Can you work these out from the model? Positions are in its coordinate system, mm. Face numbers are marked on the shaded views. Coordinates: 2 decimals unless noted, no trailing zeros. Order: outer loops, then holes, each group sorted by start corner. A loop starts at its lowest first (then second) coordinate and runs counter-clockwise, first axis right, second up. Notation, with made-up numbers: (-37.75, 32) - (21.25, 32) arc R31 ccw to (21.25, 59) - close; hole circle Ø11 at (21, -39.5). An arc over 180 degrees is marked (long way). Use a Markdown table: item, result. Add a question column.
(1) For pin 1 Ø2 at (y, z) = (14, 3) entering from -X; pin 2 Ø1.5 at (x, z) = (-14.5, 9) entering from +Y; pin 3 Ø1 at (y, z) = (25, 1.5) entering from +X; pin 4 Ø6 at (x, y) = (-40, 0) entering from +Z, each with a flat end and sliding along its axis, tell me the tip position at first contact or that it passes through.
(2) We'd pull the mould along Y, two halves only. Please class the marked faces 1, 2 and 3: pulls with the +Y half, pulls with the -Y half, needs draft (parallel to the pull), parting line crosses it, or undercut.
(3) I want a section at B-B (z = 3.25). List the corners of the cut face in (x, y) for me.
(4) If I drill on L1, parallel to X at y = -1.5, z = 3.5; L2, parallel to X at y = 39.5, z = 1; L3, parallel to X at y = 24.5, z = 4.75, over which ranges is the centre line in solid material (lowest first)? Write a range as [from, to].
(5) I want a section at A-A (x = 0). List the corners of the cut face in (y, z) for me.
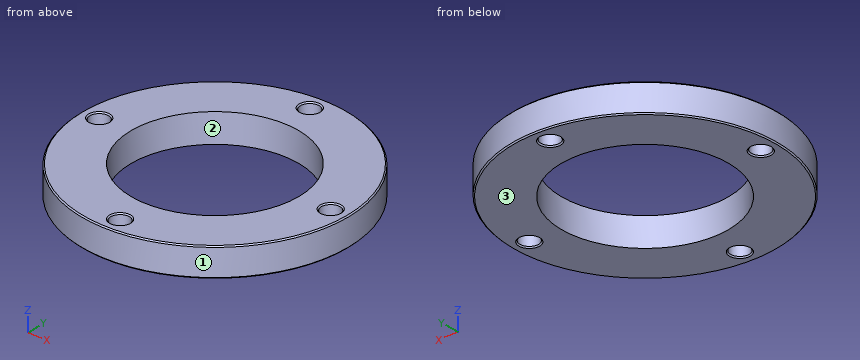
Autodesk Inventor part; units mm, degrees
ref_plane "YZ Plane" through (0, 0, 0) normal (1, 0, 0) x (0, 1, 0)
ref_plane "XZ Plane" through (0, 0, 0) normal (0, 1, 0) x (-1, 0, 0)
ref_plane "XY Plane" through (0, 0, 0) normal (0, 0, 1) x (1, 0, 0)
sketch "Sketch1" plane through (0, 0, 0) normal (0, 0, 1) x (1, 0, 0)
  circle A0 centre (0, 0) radius 46
  circle A1 centre (0, 0) radius 29
  dimension "d0" = 58
  dimension "d1" = 92
extrude "Extrusion1" add sketch "Sketch1" along normal blind 10
sketch "Sketch2" plane through (0, 0, 10) normal (0, 0, 1) x (1, 0, 0)
  circle A0 centre (0, 0) radius 29
  circle A1 centre (0, 0) radius 40 construction
  point P0 (0, 40)
  dimension "d4" = 80
hole "Hole1" at (0, 40, 10) direction (0, 0, -1) diameter 6.5 end through all
pattern_circular "Circular Pattern1" count 4 over 360 about axis through (0, 0, 0) along (0, 0, 1) of "Hole1"
chamfer "Chamfer1" distance 0.4 angle 45 10 edges at (-46, 0, 0) (-46, 0, 10) (0, 43.25, 0) (-43.25, 0, 0) (43.25, 0, 0) (0, -43.25, 0) (43.25, 0, 10) (0, 43.25, 10) (0, -43.25, 10) (-43.25, 0, 10)
equation "\"d0\" = ID"
equation "\"d1\" = OD"
equation "\"OD\" = 92"
equation "\"ID\" = 58"
properties part number "pld_flange_flat_ak"
Answers follow:
| question | item | result |
|---|---|---|
| 1 | pin 1 | stops at x = -44.12 |
| 1 | pin 2 | stops at y = 43.9 |
| 1 | pin 3 | stops at x = 38.93 |
| 1 | pin 4 | passes through |
| 2 | face 1 | parting line crosses it |
| 2 | face 2 | undercut |
| 2 | face 3 | needs draft |
| 3 | outline | circle Ø92 at (0, 0); hole circle Ø6.5 at (-40, 0); hole circle Ø58 at (0, 0); hole circle Ø6.5 at (0, -40); hole circle Ø6.5 at (0, 40); hole circle Ø6.5 at (40, 0) |
| 4 | L1 | x = [-45.98, -42.88], [-37.12, -28.96], [28.96, 37.12], [42.88, 45.98] |
| 4 | L2 | x = [-23.57, -3.21], [3.21, 23.57] |
| 4 | L3 | x = [-38.93, -15.52], [15.52, 38.93] |
| 5 | outline | (-46, 0.4) - (-45.6, 0) - (-43.65, 0) - (-43.25, 0.4) - (-43.25, 9.6) - (-43.65, 10) - (-45.6, 10) - (-46, 9.6) - close; (-36.75, 0.4) - (-36.35, 0) - (-29, 0) - (-29, 10) - (-36.35, 10) - (-36.75, 9.6) - close; (29, 0) - (36.35, 0) - (36.75, 0.4) - (36.75, 9.6) - (36.35, 10) - (29, 10) - close; (43.25, 0.4) - (43.65, 0) - (45.6, 0) - (46, 0.4) - (46, 9.6) - (45.6, 10) - (43.65, 10) - (43.25, 9.6) - close |
